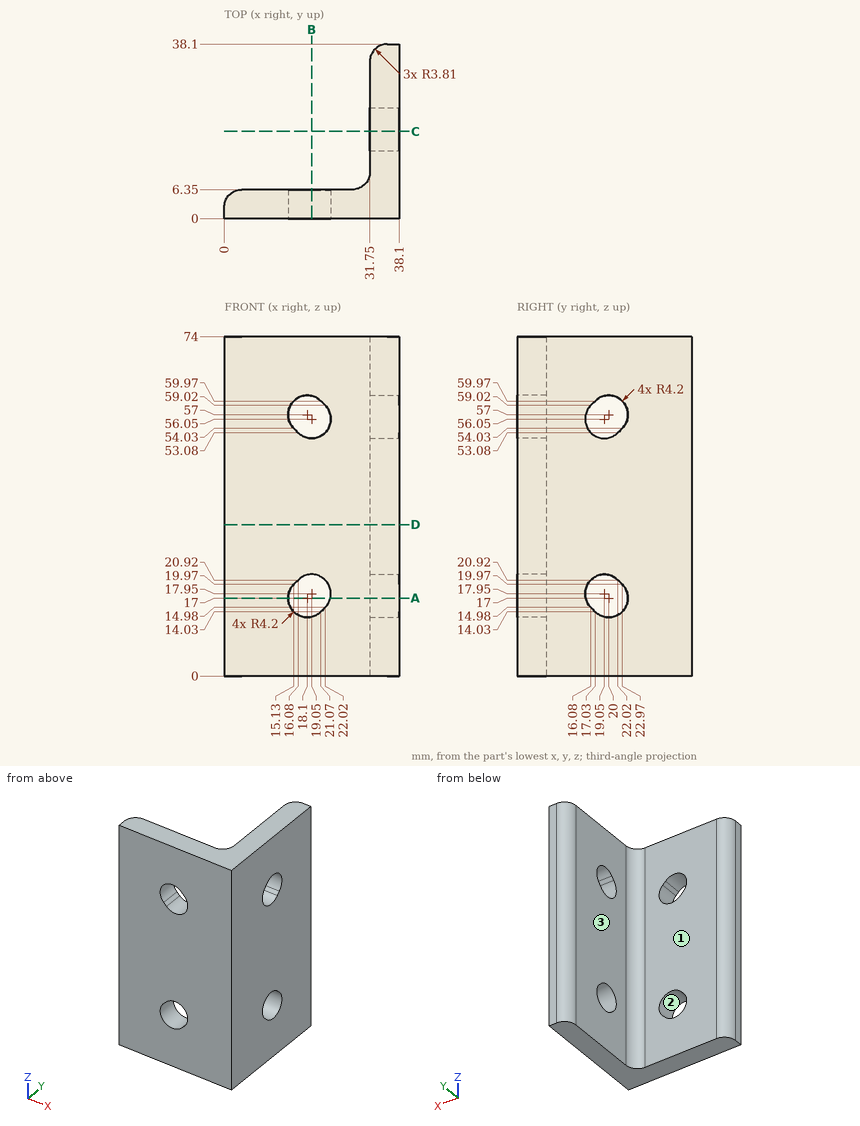
Verification items for this drawing (mm, ordinates from the low corner). Round coordinates to 2 decimals unless told otherwise and drop trailing zeros. Loops run counter-clockwise (first coordinate to the right, second up) from the corner with the lowest first, then second, coordinate; pieces in that order, holes last. Notation, with made-up numbers: (-4.75, -5) -> (6.25, -5) arc R16 ccw to (6.25, 5) -> close; hole circle Ø3 at (42.25, 45). An arc over 180 degrees is marked (long way). Write item = value, one per line. Start each with the question number.
1) Sectioned sample at B-B, the plane x = 19.05. Record the cut outline in (y, z).
2) Sectioned sample at A-A, the plane z = 17. Record the cut outline in (x, y), plus the area to 3 significant figures.
3) Thickness scan on probe 1 along Z at (x, y) = (21, 4.5); probe 2 along X at (y, z) = (22.5, 67); probe 3 along Y at (x, z) = (20, 8.5). Record the ranges inside material, lowest first.
4) Sectioned sample at D-D, the plane z = 33. Record the cut outline in (x, y), plus the area to 3 significant figures.
5) Gauge pin test, flat end, axial feed: pin 1 Ø3 at (y, z) = (27.5, 7.5) entering from -X. Record the tip position at first contact, or that the pin passes through.
6) Release check for a two-part mould opening along X. For the marked faces 1, 2 and 3 record: released by +X, released by -X, zero draft, split by the parting line, or undercut.
7) Sectioned sample at C-C, the plane y = 19.05. Record the cut outline in (x, z).
Results are:
q1.outline = (0, 0) -> (6.35, 0) -> (6.35, 12.91) -> (0, 12.91) -> close; (0, 22.15) -> (6.35, 22.15) -> (6.35, 51.85) -> (0, 51.85) -> close; (0, 61.09) -> (6.35, 61.09) -> (6.35, 74) -> (0, 74) -> close
q2.outline = (0, 0) -> (13.9, 0) -> (13.9, 6.35) -> (3.81, 6.35) arc R3.81 ccw to (0, 2.54) -> close; (23.14, 0) -> (38.1, 0) -> (38.1, 14.96) -> (31.75, 14.96) -> (31.75, 10.16) arc R3.81 cw to (27.94, 6.35) -> (23.14, 6.35) -> close; (31.75, 24.2) -> (38.1, 24.2) -> (38.1, 38.1) -> (35.56, 38.1) arc R3.81 ccw to (31.75, 34.29) -> close
q2.area = 323 mm^2
q3.probe_1 = 0 to 13.96, 21.67 to 52.33, 60.04 to 74
q3.probe_2 = 31.75 to 38.1
q3.probe_3 = 0 to 6.35
q4.outline = (0, 0) -> (38.1, 0) -> (38.1, 38.1) -> (35.56, 38.1) arc R3.81 ccw to (31.75, 34.29) -> (31.75, 10.16) arc R3.81 cw to (27.94, 6.35) -> (3.81, 6.35) arc R3.81 ccw to (0, 2.54) -> close
q4.area = 440 mm^2
q5.pin_1 = 31.75
q6.face_1 = zero draft
q6.face_2 = undercut
q6.face_3 = released by -X
q7.outline = (31.75, 0) -> (38.1, 0) -> (38.1, 12.91) -> (31.75, 12.91) -> close; (31.75, 22.15) -> (38.1, 22.15) -> (38.1, 51.85) -> (31.75, 51.85) -> close; (31.75, 61.09) -> (38.1, 61.09) -> (38.1, 74) -> (31.75, 74) -> close
